from build123d import *

# Parameters (mm, degrees)
BOSS_EXTRUDE1_DEPTH = 10
SKETCH3_R           = 6.05
SKETCH3_R_2         = 4.05
BOSS_EXTRUDE2_DEPTH = 25
SKETCH4_R           = 1.5
CUT_EXTRUDE1_DEPTH  = 113.073458053
SKETCH5_R           = 3
CUT_EXTRUDE2_DEPTH  = 4
CUT_EXTRUDE3_DEPTH  = 113.073458053
SKETCH7_W           = 85.997746486
SKETCH7_H           = 30.827207152
SKETCH7_W_2         = 81.997746486
SKETCH7_H_2         = 26.827207152
BOSS_EXTRUDE3_DEPTH = 22
SKETCH9_W           = 26.827207152
SKETCH9_H           = 22
CUT_EXTRUDE7_DEPTH  = 22
BOSS_EXTRUDE4_START = 50
BOSS_EXTRUDE4_DEPTH = 50
CUT_EXTRUDE8_DEPTH  = 22
CHAMFER2_SIZE       = 4


with BuildPart() as part:
    # Sketch2 → Boss-Extrude1 (new body)
    with BuildSketch(Plane(origin=(0, 0, 0), x_dir=(1, 0, 0), z_dir=(0, 1, 0))):
        with BuildLine():
            Line((-76.2, 63.5), (76.2, 63.5))
            ThreePointArc((76.2, 63.5), (85.180256121, 59.780256121), (88.9, 50.8))
            Line((88.9, 50.8), (88.9, -50.8))
            ThreePointArc((88.9, -50.8), (85.180256121, -59.780256121), (76.2, -63.5))
            Line((76.2, -63.5), (-76.2, -63.5))
            ThreePointArc((-76.2, -63.5), (-85.180256121, -59.780256121), (-88.9, -50.8))
            Line((-88.9, -50.8), (-88.9, 50.8))
            ThreePointArc((-88.9, 50.8), (-85.180256121, 59.780256121), (-76.2, 63.5))
        make_face()
    extrude(amount=BOSS_EXTRUDE1_DEPTH)

    # Sketch3 → Boss-Extrude2 (add)
    # profile 1 of 2: a face of its own
    with BuildSketch(Plane(origin=(0, 10, 0), x_dir=(1, 0, 0), z_dir=(0, 1, 0))):
        with Locations(Location((0, 48, 0), (0, 0, 270))):
            Circle(SKETCH3_R)
        with Locations(Location((0, 48, 0), (0, 0, 270))):
            Circle(SKETCH3_R_2, mode=Mode.SUBTRACT)
    # profile 2 of 2: a face of its own
    with BuildSketch(Plane(origin=(0, 10, 0), x_dir=(1, 0, 0), z_dir=(0, 1, 0))):
        with Locations(Location((0, -48.5, 0), (0, 0, 270))):
            Circle(SKETCH3_R)
        with Locations(Location((0, -48.5, 0), (0, 0, 270))):
            Circle(SKETCH3_R_2, mode=Mode.SUBTRACT)
    extrude(amount=BOSS_EXTRUDE2_DEPTH)

    # Sketch4 → Cut-Extrude1 (cut, through all)
    with BuildSketch(Plane(origin=(0, 10, 0), x_dir=(1, 0, 0), z_dir=(0, 1, 0))):
        with Locations(Location((-78.23, 10.69, 0), (0, 0, 270))):
            Circle(SKETCH4_R)
        with Locations(Location((-78.23, -10.69, 0), (0, 0, 270))):
            Circle(SKETCH4_R)
        with Locations(Location((78.23, -10.69, 0), (0, 0, 90))):
            Circle(SKETCH4_R)
        with Locations(Location((78.23, 10.69, 0), (0, 0, 90))):
            Circle(SKETCH4_R)
    extrude(amount=-CUT_EXTRUDE1_DEPTH, mode=Mode.SUBTRACT)

    # Sketch5 → Cut-Extrude2 (cut)
    with BuildSketch(Plane.XZ):
        with Locations(Location((-78.23, 10.69, 0), (0, 0, 270))):
            Circle(SKETCH5_R)
        with Locations(Location((-78.23, -10.69, 0), (0, 0, 270))):
            Circle(SKETCH5_R)
        with Locations(Location((78.23, 10.69, 0), (0, 0, 270))):
            Circle(SKETCH5_R)
        with Locations(Location((78.23, -10.69, 0), (0, 0, 270))):
            Circle(SKETCH5_R)
    extrude(amount=-CUT_EXTRUDE2_DEPTH, mode=Mode.SUBTRACT)

    # Sketch6 → Cut-Extrude3 (cut, through all)
    with BuildSketch(Plane(origin=(0, 10, 0), x_dir=(1, 0, 0), z_dir=(0, 1, 0))):
        with BuildLine():
            Line((-43, 8.5), (43, 8.5))
            ThreePointArc((43, 8.5), (45.828427125, 7.328427125), (47, 4.5))
            Line((47, 4.5), (47, -4.5))
            ThreePointArc((47, -4.5), (45.828427125, -7.328427125), (43, -8.5))
            Line((43, -8.5), (-43, -8.5))
            ThreePointArc((-43, -8.5), (-45.828427125, -7.328427125), (-47, -4.5))
            Line((-47, -4.5), (-47, 4.5))
            ThreePointArc((-47, 4.5), (-45.828427125, 7.328427125), (-43, 8.5))
        make_face()
    extrude(amount=-CUT_EXTRUDE3_DEPTH, mode=Mode.SUBTRACT)

    # Sketch7 → Boss-Extrude3 (add)
    with BuildSketch(Plane(origin=(0, 10, 0), x_dir=(1, 0, 0), z_dir=(0, 1, 0))):
        with Locations((-0.001126757, -23.913603576)):
            Rectangle(SKETCH7_W, SKETCH7_H)
        with Locations((-0.001126757, -23.913603576)):
            Rectangle(SKETCH7_W_2, SKETCH7_H_2, mode=Mode.SUBTRACT)
    extrude(amount=BOSS_EXTRUDE3_DEPTH)

    # Sketch9 → Cut-Extrude7 (cut)
    with BuildSketch(Plane.ZY.offset(43)):
        with Locations((23.913603576, 21)):
            Rectangle(SKETCH9_W, SKETCH9_H)
    extrude(amount=-CUT_EXTRUDE7_DEPTH, mode=Mode.SUBTRACT)

    # Sketch10 → Boss-Extrude4 (add)
    with BuildSketch(Plane(origin=(0, 10, 0), x_dir=(1, 0, 0), z_dir=(0, 1, 0)).offset(BOSS_EXTRUDE4_START)):
        with BuildLine():
            Line((-49, 4.5), (-49, -4.5))
            ThreePointArc((-49, -4.5), (-47.242640687, -8.742640687), (-43, -10.5))
            Line((-43, -10.5), (-43, -8.5))
            ThreePointArc((-43, -8.5), (-45.828427125, -7.328427125), (-47, -4.5))
            Line((-47, -4.5), (-47, 4.5))
            ThreePointArc((-47, 4.5), (-45.828427125, 7.328427125), (-43, 8.5))
            Line((-43, 8.5), (43, 8.5))
            ThreePointArc((43, 8.5), (45.828427125, 7.328427125), (47, 4.5))
            Line((47, 4.5), (47, -4.5))
            ThreePointArc((47, -4.5), (45.828427125, -7.328427125), (43, -8.5))
            Line((43, -8.5), (43, -10.5))
            ThreePointArc((43, -10.5), (47.242640687, -8.742640687), (49, -4.5))
            Line((49, -4.5), (49, 4.5))
            ThreePointArc((49, 4.5), (47.242640687, 8.742640687), (43, 10.5))
            Line((43, 10.5), (-43, 10.5))
            ThreePointArc((-43, 10.5), (-47.242640687, 8.742640687), (-49, 4.5))
        make_face()
    extrude(amount=-BOSS_EXTRUDE4_DEPTH)

    # Sketch11 → Cut-Extrude8 (cut)
    with BuildSketch(Plane.XZ):
        with BuildLine():
            Line((-17.302391978, 25.904152562), (17.302391978, 25.904152562))
            ThreePointArc((17.302391978, 25.904152562), (19.873033072, 23.333511468), (17.302391978, 20.762870374))
            Line((17.302391978, 20.762870374), (-17.302391978, 20.762870374))
            ThreePointArc((-17.302391978, 20.762870374), (-19.873033072, 23.333511468), (-17.302391978, 25.904152562))
        make_face()
    extrude(amount=-CUT_EXTRUDE8_DEPTH, mode=Mode.SUBTRACT)

    # Chamfer2
    # the kernel refuses this chamfer: 4 mm, written as the material it adds along each edge
    with BuildSketch(Plane(origin=(0, 10, -48), x_dir=(0, 0, 1), z_dir=(-1, 0, 0))) as chamfer2_piece_1:
        Polygon((6.05 + CHAMFER2_SIZE, 0), (6.05, CHAMFER2_SIZE), (6.05, 0), align=None)
    revolve(axis=Axis((0, 10, -48), (0, 1, 0)))
    with BuildSketch(Plane(origin=(0, 10, 48.5), x_dir=(0, 0, 1), z_dir=(-1, 0, 0))) as chamfer2_piece_2:
        Polygon((6.05 + CHAMFER2_SIZE, 0), (6.05, CHAMFER2_SIZE), (6.05, 0), align=None)
    revolve(axis=Axis((0, 10, 48.5), (0, 1, 0)))


solid = part.part
The listing builds one solid part. Answer for the finished solid, in the listing's coordinates (mm). A direction names the side the tool comes from. Round coordinates to 2 decimals unless told otherwise and drop trailing zeros. Order: outer loops, then holes, each group sorted by start corner. A loop starts at its lowest first (then second) coordinate and runs counter-clockwise, first axis right, second up. Notation, with made-up numbers: (68, 24) -> (104, 24) arc R25 cw to (104, 61) -> close; hole circle Ø4 at (87, 9.25). An arc over 180 degrees is marked (long way). One line per item, written item: value.
Item 1: Given P1, Ø5, axis at y = 33.5, z = 4, coming from the +X side; P2, Ø11, axis at x = -13, y = 23, coming from the +Z side; P3, Ø12, axis at x = -40.5, y = 19, coming from the -Z side, each flat-ended and moving along its own axis, determine where each tip first touches the part or whether it passes through.
Taken from the geometry:
P1: stops at x = 49
P2: stops at z = 39.33
P3: stops at z = -10.5
Item 2: Find section A-A, the plane y = 24.5. Give the vertices of the cut face in (x, z).
Taken from the geometry:
outline: (-49, -4.5) arc R6 ccw to (-43, -10.5) -> (43, -10.5) arc R6 ccw to (49, -4.5) -> (49, 4.5) arc R6 ccw to (43, 10.5) -> (43, 8.5) arc R4 cw to (47, 4.5) -> (47, -4.5) arc R4 cw to (43, -8.5) -> (-43, -8.5) arc R4 cw to (-47, -4.5) -> (-47, 4.5) arc R4 cw to (-43, 8.5) -> (43, 8.5) -> (43, 39.33) -> (-43, 39.33) -> (-43, 37.33) -> (41, 37.33) -> (41, 10.5) -> (-43, 10.5) arc R6 ccw to (-49, 4.5) -> close; circle Ø12.1 at (0, -48); circle Ø12.1 at (0, 48.5); hole circle Ø8.1 at (0, -48); hole circle Ø8.1 at (0, 48.5)
Item 3: Straight lines are drawn through the part: L1, parallel to X at y = 0.95, z = 10.69; L2, parallel to Z at x = -33, y = 26.5; L3, parallel to X at y = 6, z = -10. For each, find the intervals that lie inside material, in ascending order.
Taken from the geometry:
L1: x = -88.9 to -81.23, -75.23 to 75.23, 81.23 to 88.9
L2: z = -10.5 to -8.5, 8.5 to 10.5, 37.33 to 39.33
L3: x = -88.9 to -79.56, -76.9 to 76.9, 79.56 to 88.9
Item 4: Find section C-C, the plane y = 49. Give the vertices of the cut face in (x, z).
Taken from the geometry:
outline: (-49, -4.5) arc R6 ccw to (-43, -10.5) -> (43, -10.5) arc R6 ccw to (49, -4.5) -> (49, 4.5) arc R6 ccw to (43, 10.5) -> (43, 8.5) arc R4 cw to (47, 4.5) -> (47, -4.5) arc R4 cw to (43, -8.5) -> (-43, -8.5) arc R4 cw to (-47, -4.5) -> (-47, 4.5) arc R4 cw to (-43, 8.5) -> (-43, 10.5) arc R6 ccw to (-49, 4.5) -> close
Item 5: For faces 1 (the cylindrical face through (-47.289, 35.35, 8.696)), 2 (the flat face through (-4, 35, 50)), 3 (the cylindrical face through (45.797, 30.42, -7.359)), determine the directions among +Z, -Z, +X, -X, +Y, -Y from which every point of the face is accessible in a straight line to the end or side of a thin tool.
Taken from the geometry:
face 1: +Z, -X, +Y
face 2: +Z, +X, -X, +Y
face 3: +Y, -Y
Item 6: Find section D-D, the plane z = -48. Give the vertices of the cut face in (x, y).
Taken from the geometry:
outline: (-88.9, 0) -> (88.9, 0) -> (88.9, 10) -> (10.05, 10) -> (6.05, 14) -> (6.05, 35) -> (4.05, 35) -> (4.05, 10) -> (-4.05, 10) -> (-4.05, 35) -> (-6.05, 35) -> (-6.05, 14) -> (-10.05, 10) -> (-88.9, 10) -> close
Item 7: Find section B-B, the plane x = -40. Give the vertices of the cut face in (y, z), then the cut area to 3 significant figures.
Taken from the geometry:
outline: (0, -63.5) -> (10, -63.5) -> (10, -10.5) -> (60, -10.5) -> (60, -8.5) -> (0, -8.5) -> close; (0, 8.5) -> (32, 8.5) -> (32, 10.5) -> (10, 10.5) -> (10, 37.33) -> (32, 37.33) -> (32, 39.33) -> (10, 39.33) -> (10, 63.5) -> (0, 63.5) -> close
area: 1,290 mm2
Item 8: For a pull along Z with two mould halves and no side action, classify faces 4 (the cylindrical face through (0.266, 24.353, 42.456)), 5 (the flat face through (49, 35, 0)), 6 (the flat face through (1, 5, 63.5)) as released by +Z, released by -Z, zero draft, split by the parting line, or undercut.
Taken from the geometry:
face 4: undercut
face 5: zero draft
face 6: released by +Z
